Source: CAD feature listing. Evaluate the final solid. Frame: model axes, mm. Give positions to 0.01 mm unless a question says otherwise; leave off trailing zeros. Order: outer loops, then holes, each group sorted by start corner. A loop starts at its lowest first (then second) coordinate and runs counter-clockwise, first axis right, second up.
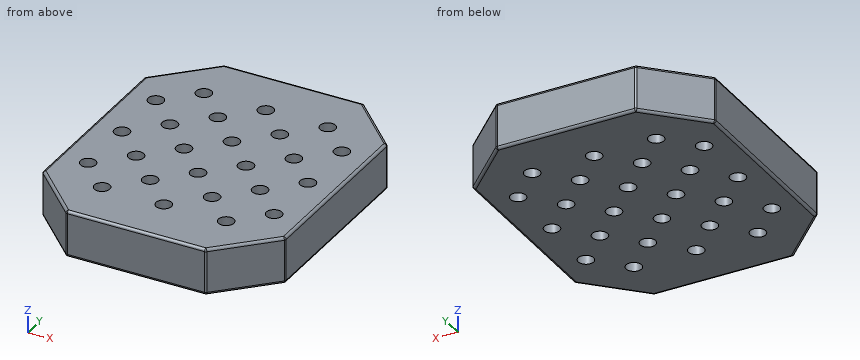
from build123d import *

# Parameters (mm, degrees)
SKETCH_W     = 94
SKETCH_H     = 112
SKETCH_R     = 3
PAD_DEPTH    = 18
POCKET_DEPTH = 18.001
FILLET_R     = 1
FILLET001_R  = 1
FILLET002_R  = 1
FILLET003_R  = 1


with BuildPart() as part:
    # Sketch → Pad (new body)
    with BuildSketch(Plane.XY):
        with Locations((-47, 56)):
            Rectangle(SKETCH_W, SKETCH_H)
        with Locations((-47, 19.7281)):
            Circle(SKETCH_R, mode=Mode.SUBTRACT)
        with Locations((-23, 68)):
            Circle(SKETCH_R, mode=Mode.SUBTRACT)
        with Locations((-23, 44)):
            Circle(SKETCH_R, mode=Mode.SUBTRACT)
        with Locations((-23, 20)):
            Circle(SKETCH_R, mode=Mode.SUBTRACT)
        with Locations((-23, 92)):
            Circle(SKETCH_R, mode=Mode.SUBTRACT)
        with Locations((-47, 44)):
            Circle(SKETCH_R, mode=Mode.SUBTRACT)
        with Locations((-47, 68)):
            Circle(SKETCH_R, mode=Mode.SUBTRACT)
        with Locations((-47, 92)):
            Circle(SKETCH_R, mode=Mode.SUBTRACT)
        with Locations((-71, 92)):
            Circle(SKETCH_R, mode=Mode.SUBTRACT)
        with Locations((-71, 68)):
            Circle(SKETCH_R, mode=Mode.SUBTRACT)
        with Locations((-59, 32)):
            Circle(SKETCH_R, mode=Mode.SUBTRACT)
        with Locations((-71, 19.92972)):
            Circle(SKETCH_R, mode=Mode.SUBTRACT)
        with Locations((-71, 44)):
            Circle(SKETCH_R, mode=Mode.SUBTRACT)
        with Locations((-59, 56)):
            Circle(SKETCH_R, mode=Mode.SUBTRACT)
        with Locations((-35, 56)):
            Circle(SKETCH_R, mode=Mode.SUBTRACT)
        with Locations((-35, 32)):
            Circle(SKETCH_R, mode=Mode.SUBTRACT)
        with Locations((-35, 80)):
            Circle(SKETCH_R, mode=Mode.SUBTRACT)
        with Locations((-59, 80)):
            Circle(SKETCH_R, mode=Mode.SUBTRACT)
        with Locations((-83, 32)):
            Circle(SKETCH_R, mode=Mode.SUBTRACT)
        with Locations((-83, 56)):
            Circle(SKETCH_R, mode=Mode.SUBTRACT)
        with Locations((-83, 80)):
            Circle(SKETCH_R, mode=Mode.SUBTRACT)
        with Locations((-11, 80)):
            Circle(SKETCH_R, mode=Mode.SUBTRACT)
        with Locations((-11, 56)):
            Circle(SKETCH_R, mode=Mode.SUBTRACT)
        with Locations((-11, 32)):
            Circle(SKETCH_R, mode=Mode.SUBTRACT)
    extrude(amount=PAD_DEPTH)

    # Sketch001 (on Face30 of Pad) → Pocket (cut, through all)
    with BuildSketch(Plane.XY.offset(18)):
        Polygon((0, 0), (0, 20), (-20, 0), align=None)
        Polygon((0, 112), (0, 92), (-20, 112), align=None)
        Polygon((-74, 112), (-94, 112), (-94, 92), align=None)
        Polygon((-94, 20), (-94, 0), (-74, 0), align=None)
    extrude(amount=-POCKET_DEPTH, mode=Mode.SUBTRACT)

    # Fillet
    fillet_edges = [part.edges().sort_by_distance(p)[0] for p in [
        (-84, 102, 18),
        (-47, 112, 18),
        (-10, 102, 18),
        (0, 56, 18),
        (-10, 10, 18),
        (-47, 0, 18),
        (-84, 10, 18),
        (-94, 56, 18),
    ]]
    fillet(fillet_edges, radius=FILLET_R)

    # Fillet001
    fillet001_edges = [part.edges().sort_by_distance(p)[0] for p in [
        (0, 20, 8.5),
        (-20, 0, 8.5),
        (0, 92, 8.5),
        (-20, 112, 8.5),
    ]]
    fillet(fillet001_edges, radius=FILLET001_R)

    # Fillet002
    fillet002_edges = [part.edges().sort_by_distance(p)[0] for p in [
        (-74, 112, 8.5),
        (-94, 92, 8.5),
        (-94, 20, 8.5),
        (-74, 0, 8.5),
    ]]
    fillet(fillet002_edges, radius=FILLET002_R)

    # Fillet003
    fillet003_edges = [part.edges().sort_by_distance(p)[0] for p in [
        (-47, 112, 0),
        (-84, 102, 0),
        (-94, 56, 0),
        (-84, 10, 0),
        (-47, 0, 0),
        (-10, 10, 0),
        (0, 56, 0),
        (-10, 102, 0),
    ]]
    fillet(fillet003_edges, radius=FILLET003_R)


solid = part.part
1) Section query C-C on x = -71. Output: boundary loops of the cut face in (y, z), and give its area (3 significant figures).
Checks:
outline: (0, 1) arc R1 ccw to (1, 0) - (16.93, 0) - (16.93, 18) - (1, 18) arc R1 ccw to (0, 17) - close; (22.93, 0) - (41, 0) - (41, 18) - (22.93, 18) - close; (47, 0) - (65, 0) - (65, 18) - (47, 18) - close; (71, 0) - (89, 0) - (89, 18) - (71, 18) - close; (95, 0) - (111, 0) arc R1 ccw to (112, 1) - (112, 17) arc R1 ccw to (111, 18) - (95, 18) - close
area: 1,580 mm2
2) First-contact query: pin 1 Ø1 at (x, z) = (-75, 12) entering from -Y; pin 2 Ø5.5 at (x, y) = (-47, 92) entering from -Z. Flat tips, straight axial feed; report the tip coordinate or a pass-through.
Checks:
pin 1: stops at y = 0.5
pin 2: passes through
3) Ray query, L1, parallel to Y at x = -47, z = 12.5; L2, parallel to Y at x = -35, z = 5.25; L3, parallel to Y at x = -71, z = 7.5. Return the intervals inside material, ascending.
Checks:
L1: y = 0 to 16.73, 22.73 to 41, 47 to 65, 71 to 89, 95 to 112
L2: y = 0 to 29, 35 to 53, 59 to 77, 83 to 112
L3: y = 0 to 16.93, 22.93 to 41, 47 to 65, 71 to 89, 95 to 112
4) Section query D-D on z = 4.75. State how many separate pieces and enclosed holes the cut face has, and give its area (3 significant figures).
Checks:
separate pieces: 1
enclosed holes: 24
area: 9,050 mm2
5) Section query A-A on x = -59. Output: boundary loops of the cut face in (y, z), and give its area (3 significant figures).
Checks:
outline: (0, 1) arc R1 ccw to (1, 0) - (29, 0) - (29, 18) - (1, 18) arc R1 ccw to (0, 17) - close; (35, 0) - (53, 0) - (53, 18) - (35, 18) - close; (59, 0) - (77, 0) - (77, 18) - (59, 18) - close; (83, 0) - (111, 0) arc R1 ccw to (112, 1) - (112, 17) arc R1 ccw to (111, 18) - (83, 18) - close
area: 1,690 mm2
6) Section query B-B on y = 80. Output: boundary loops of the cut face in (x, z), and give its area (3 significant figures).
Checks:
outline: (-94, 1) arc R1 ccw to (-93, 0) - (-86, 0) - (-86, 18) - (-93, 18) arc R1 ccw to (-94, 17) - close; (-80, 0) - (-62, 0) - (-62, 18) - (-80, 18) - close; (-56, 0) - (-38, 0) - (-38, 18) - (-56, 18) - close; (-32, 0) - (-14, 0) - (-14, 18) - (-32, 18) - close; (-8, 0) - (-1, 0) arc R1 ccw to (0, 1) - (0, 17) arc R1 ccw to (-1, 18) - (-8, 18) - close
area: 1,260 mm2
